```python
from build123d import *

# Parameters (mm, degrees)
SKETCH1_W           = 88.9
SKETCH1_H           = 12.7
BOSS_EXTRUDE1_DEPTH = 6.35
SKETCH3_R           = 1.729482421
SKETCH3_R_2         = 1.816224302
CUT_EXTRUDE1_DEPTH  = 6.35


with BuildPart() as part:
    # Sketch1 → Boss-Extrude1 (new body)
    with BuildSketch(Plane.XY):
        with Locations((34.234782609, 12.285869565)):
            Rectangle(SKETCH1_W, SKETCH1_H)
    extrude(amount=BOSS_EXTRUDE1_DEPTH)

    # Sketch3 → Cut-Extrude1 (cut)
    with BuildSketch(Plane.XY.offset(6.35)):
        with Locations((21.534782609, 12.285869565)):
            Circle(SKETCH3_R)
        with Locations((-3.865217391, 12.285869565)):
            Circle(SKETCH3_R_2)
        with BuildLine():
            Line((55.824782609, 14.825869565), (72.741182609, 14.825869565))
            ThreePointArc((72.741182609, 14.825869565), (75.281182609, 12.285869565), (72.741182609, 9.745869565))
            Line((72.741182609, 9.745869565), (55.824782609, 9.745869565))
            ThreePointArc((55.824782609, 9.745869565), (53.284782609, 12.285869565), (55.824782609, 14.825869565))
        make_face()
        with BuildLine():
            Line((47.341182609, 9.745869565), (30.424782609, 9.745869565))
            ThreePointArc((30.424782609, 9.745869565), (27.884782609, 12.285869565), (30.424782609, 14.825869565))
            Line((30.424782609, 14.825869565), (47.341182609, 14.825869565))
            ThreePointArc((47.341182609, 14.825869565), (49.881182609, 12.285869565), (47.341182609, 9.745869565))
        make_face()
    extrude(amount=-CUT_EXTRUDE1_DEPTH, mode=Mode.SUBTRACT)


solid = part.part
```
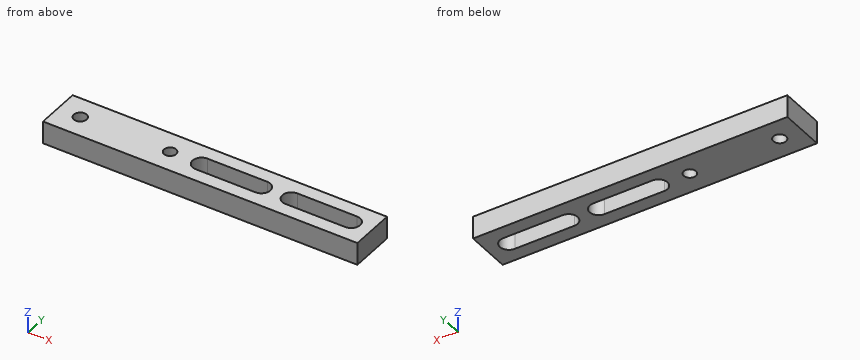
Read the model definition and answer for the solid it produces. Units are mm, in the model's axes. Round coordinates to 2 decimals unless told otherwise and drop trailing zeros. Write each loop counter-clockwise with the first axis right and the second up, starting at its lowest first coordinate (ties: lowest second). Pieces come first, ordered by that corner, then holes. Notation, with made-up numbers: (40.25, -24.5) - (91.25, -24.5) arc R21 cw to (91.25, 6.5) - close; hole circle Ø2 at (31.5, 25). An arc over 180 degrees is marked (long way). One line per item, written item: value.
Q1. Find section B-B (z = 3.75). Determine the outline of the cut face in (x, y), and give its area (3 significant figures).
The answers:
outline: (-10.22, 5.94) - (78.68, 5.94) - (78.68, 18.64) - (-10.22, 18.64) - close; hole circle Ø3.63 at (-3.87, 12.29); hole circle Ø3.46 at (21.53, 12.29); hole (30.42, 9.75) - (47.34, 9.75) arc R2.54 ccw to (47.34, 14.83) - (30.42, 14.83) arc R2.54 ccw to start; hole (55.82, 9.75) - (72.74, 9.75) arc R2.54 ccw to (72.74, 14.83) - (55.82, 14.83) arc R2.54 ccw to start
area: 897 mm2
Q2. Straight lines are drawn through the part: line 1 (Y direction, x = 33, z = 6.25); line 2 (X direction, y = 12, z = 0.75); line 3 (X direction, y = 11.5, z = 1.25). For each, find the intervals that lie inside material, in ascending order. Write a range as from..to.
The answers:
line 1: y = 5.94..9.75, 14.83..18.64
line 2: x = -10.22..-5.66, -2.07..19.83, 23.24..27.9, 49.87..53.3, 75.27..78.68
line 3: x = -10.22..-5.5, -2.23..19.99, 23.08..28.01, 49.76..53.41, 75.16..78.68
Q3. Find section A-A (x = 70). Determine the outline of the cut face in (y, z), and give its area (3 significant figures).
The answers:
outline: (5.94, 0) - (9.75, 0) - (9.75, 6.35) - (5.94, 6.35) - close; (14.83, 0) - (18.64, 0) - (18.64, 6.35) - (14.83, 6.35) - close
area: 48.4 mm2
